Autodesk Inventor part; units mm, degrees
ref_plane "YZ Plane" through (0, 0, 0) normal (1, 0, 0) x (0, 1, 0)
ref_plane "XZ Plane" through (0, 0, 0) normal (0, 1, 0) x (-1, 0, 0)
ref_plane "XY Plane" through (0, 0, 0) normal (0, 0, 1) x (1, 0, 0)
sketch "スケッチ1" plane through (0, 0, 0) normal (0, 1, 0) x (-1, 0, 0)
  line L0 (0, 0) -> (-9, 0)
  line L1 (-9, 0) -> (-9, -9)
  line L2 (-9, -9) -> (0, -9)
  line L3 (0, -9) -> (0, 0)
  line L4 (-1.2, -1.2) -> (-7.8, -1.2)
  line L5 (-7.8, -1.2) -> (-7.8, -7.8)
  line L6 (-7.8, -7.8) -> (-1.2, -7.8)
  line L7 (-1.2, -7.8) -> (-1.2, -1.2)
  dimension "d0" = 9
  dimension "d1" = 9
  dimension "d2" = 6.6
  dimension "d3" = 6.6
  dimension "d4" = 1.2
  dimension "d5" = 1.2
extrude "押し出し1" add sketch "スケッチ1" along normal blind 18
sketch "スケッチ2" plane through (0, 0, 0) normal (0, 0, 1) x (1, 0, 0)
  line L0 (0, 0) -> (9, 0)
  line L1 (7.8, 0) -> (7.8, 18)
  line L2 (9, 0) -> (9, 18)
  point P0 (4.5, 4.5)
  dimension "d8" = 4.5
  dimension "d26" = 4.5
hole "穴1" at (4.5, 4.5, 0) direction (0, 0, -1) diameter 3 end through all
sketch "スケッチ3" plane through (9, 0, 0) normal (1, 0, 0) x (0, 0, -1)
  line L0 (0, 18) -> (9, 18)
  line L1 (0, 0) -> (0, 18)
  point P0 (4.5, 13.5)
  dimension "d17" = 4.5
  dimension "d18" = 4.5
hole "穴2" at (9, 13.5, -4.5) direction (-1, 0, 0) diameter 3 end through all
sketch "スケッチ4" plane through (0, 0, 0) normal (0, 0, 1) x (1, 0, 0)
  line L0 (0, 18) -> (9, 18)
  line L1 (0, 0) -> (0, 18)
  point P0 (4.5, 13.5)
  dimension "d27" = 4.5
  dimension "d28" = 4.5
hole "穴3" at (4.5, 13.5, 0) direction (0, 0, -1) diameter 5 end through all
sketch "スケッチ5" plane through (0, 0, -9) normal (-1, 0, 0) x (0, 0, 1)
  line L0 (0, 0) -> (9, 0)
  line L1 (0, 0) -> (0, 18)
  point P0 (4.5, 4.5)
  dimension "d36" = 4.5
  dimension "d37" = 4.5
hole "穴4" at (0, 4.5, -4.5) direction (1, 0, 0) diameter 5 end through all
equation "\"d5\" = d4"
properties part number "ハンド9x9_5" material "アルミニウム 6061"
Geometry check sheet. Reference: the model listing, model coordinates, mm. A direction names the side the tool comes from. Give positions to 0.01 mm unless a question says otherwise; leave off trailing zeros. Write each loop counter-clockwise with the first axis right and the second up, starting at its lowest first coordinate (ties: lowest second). Pieces come first, ordered by that corner, then holes. Notation, with made-up numbers: (-38, 10.5) - (11, 10.5) arc R26 ccw to (11, 47.5) - close; hole circle Ø11 at (-13.75, -15). An arc over 180 degrees is marked (long way). Put each result on its own line as item: value.
1. Sectioned sample at B-B, the plane z = -4.5. Enter the section's corners in (x, y).
Ans:
outline: (0, 0) - (1.2, 0) - (1.2, 2) - (0, 2) - close; (0, 7) - (1.2, 7) - (1.2, 12) - (0, 12) - close; (0, 15) - (1.2, 15) - (1.2, 18) - (0, 18) - close; (7.8, 0) - (9, 0) - (9, 2) - (7.8, 2) - close; (7.8, 7) - (9, 7) - (9, 12) - (7.8, 12) - close; (7.8, 15) - (9, 15) - (9, 18) - (7.8, 18) - close
2. Sectioned sample at D-D, the plane x = 4.5. Enter the section's corners in (y, z).
Ans:
outline: (0, -9) - (3, -9) - (3, -7.8) - (0, -7.8) - close; (0, -1.2) - (3, -1.2) - (3, 0) - (0, 0) - close; (6, -9) - (11, -9) - (11, -7.8) - (6, -7.8) - close; (6, -1.2) - (11, -1.2) - (11, 0) - (6, 0) - close; (16, -9) - (18, -9) - (18, -7.8) - (16, -7.8) - close; (16, -1.2) - (18, -1.2) - (18, 0) - (16, 0) - close
3. Draft check along Y on faces 3 (the flat face through (1, 0, -4)), 4 (the flat face through (4, 9, 0)), 5 (the cylindrical face through (4.4, 16, -0.6)). Enter one of: +Y half, -Y half, draft (parallel to the pull), parting line (faces both ways), or undercut.
Ans:
face 3: -Y half
face 4: draft
face 5: undercut
4. Go/stop test with a flat-tipped pin: pin 1 (2.5 mm diameter, centred on y = 13.5, z = -4.5, fed in from +X). Record where the tip stops, or that it passes through.
Ans:
pin 1: passes through
5. Set-up check for faces 1 (the flat face through (1.2, 9, -5)), 2 (the cylindrical face through (3.49, 5.61, -8.41)): record each of +Z, -Z, +X, -X, +Y, -Y from which the full face is reachable in a straight line by a thin tool's end or side.
Ans:
face 1: +Y, -Y
face 2: +Z, -Z
6. Thickness scan on line 1 (Y direction, x = 8.25, z = -4.5); line 2 (Y direction, x = 4.5, z = -0.7); line 3 (Z direction, x = 6.5, y = 8.75). Record the ranges inside material, lowest first.
Ans:
line 1: y = 0 to 2, 7 to 12, 15 to 18
line 2: y = 0 to 3, 6 to 11, 16 to 18
line 3: z = -9 to -7.8, -1.2 to 0
7. Sectioned sample at A-A, the plane y = 4.5. Enter the section's corners in (x, z), plus the area to 3 significant figures.
Ans:
outline: (0, -9) - (3, -9) - (3, -7.8) - (1.2, -7.8) - (1.2, -7) - (0, -7) - close; (0, -2) - (1.2, -2) - (1.2, -1.2) - (3, -1.2) - (3, 0) - (0, 0) - close; (6, -9) - (9, -9) - (9, -7) - (7.8, -7) - (7.8, -7.8) - (6, -7.8) - close; (6, -1.2) - (7.8, -1.2) - (7.8, -2) - (9, -2) - (9, 0) - (6, 0) - close
area: 18.2 mm²
8. Sectioned sample at C-C, the plane z = -1.5. Enter the section's corners in (x, y), plus the area to 3 significant figures.
Ans:
outline: (0, 0) - (1.2, 0) - (1.2, 18) - (0, 18) - close; (7.8, 0) - (9, 0) - (9, 18) - (7.8, 18) - close
area: 43.2 mm²
